```python
from build123d import *

# Parameters (mm, degrees)
SKETCH1_3_W         = 30
SKETCH1_3_H         = 31.716112931
SKETCH1_3_W_2       = 26.4
SKETCH1_3_H_2       = 26.4
BOSS_EXTRUDE3_DEPTH = 20
SKETCH1_10_W        = 26.4
SKETCH1_10_H        = 26.4
SKETCH1_10_R        = 10.5
BOSS_EXTRUDE7_DEPTH = 5
SKETCH1_R           = 10.5
CUT_EXTRUDE1_DEPTH  = 2
SKETCH2_R           = 1.4
CUT_EXTRUDE2_DEPTH  = 15


with BuildPart() as part:
    # Sketch1_3 → Boss-Extrude3 (new body)
    # profile 1 of 3: a face of its own
    with BuildSketch(Plane.XY):
        Polygon((-189.640703899, -24.770069728), (-175.564173506, -70.171428571), (-156.564173506, -70.171428571), (-159.640703899, -23.131847808), (-159.640703899, -1.887541502), (-189.640703899, -1.887541502), align=None)
    # profile 2 of 3: a face of its own
    with BuildSketch(Plane.XY):
        Polygon((-189.640703899, -24.770069728), (-175.564173506, -70.171428571), (-156.564173506, -70.171428571), (-159.640703899, -23.131847808), (-159.640703899, -1.887541502), (-189.640703899, -1.887541502), align=None)
    # profile 3 of 3: a face of its own
    with BuildSketch(Plane.XY):
        with Locations((-174.640703899, 13.970514963)):
            Rectangle(SKETCH1_3_W, SKETCH1_3_H)
        with Locations((-174.640703899, 14.828571429)):
            Rectangle(SKETCH1_3_W_2, SKETCH1_3_H_2, mode=Mode.SUBTRACT)
    extrude(amount=-BOSS_EXTRUDE3_DEPTH)

    # Sketch1_10 → Boss-Extrude7 (add)
    # profile 1 of 2: a face of its own
    with BuildSketch(Plane.XY):
        with Locations((-174.640703899, 14.828571429)):
            Rectangle(SKETCH1_10_W, SKETCH1_10_H)
        with Locations((-174.640703899, 14.828571429)):
            Circle(SKETCH1_10_R, mode=Mode.SUBTRACT)
    # profile 2 of 2: a face of its own
    with BuildSketch(Plane.XY):
        with Locations((-174.640703899, 14.828571429)):
            Circle(SKETCH1_10_R)
        with BuildLine():
            Line((-171.403251306, 11.018203899), (-167.861898306, 7.4768509))
            ThreePointArc((-167.861898306, 7.4768509), (-174.687644898, 4.828681602), (-181.488229417, 7.540814964))
            Line((-181.488229417, 7.540814964), (-177.949263698, 11.079780683))
            ThreePointArc((-177.949263698, 11.079780683), (-179.638278417, 14.672850745), (-178.176237805, 18.364105335))
            Line((-178.176237805, 18.364105335), (-177.949263698, 18.638938958))
            Line((-177.949263698, 18.638938958), (-181.456415012, 22.146090272))
            ThreePointArc((-181.456415012, 22.146090272), (-174.665862261, 24.828539781), (-167.861898306, 22.180291958))
            Line((-167.861898306, 22.180291958), (-171.403251306, 18.638938958))
            ThreePointArc((-171.403251306, 18.638938958), (-169.640703899, 14.828571429), (-171.403251306, 11.018203899))
        make_face(mode=Mode.SUBTRACT)
    extrude(amount=-BOSS_EXTRUDE7_DEPTH)

    # Sketch1 → Cut-Extrude1 (cut)
    with BuildSketch(Plane.XY):
        with Locations((-174.640703899, 14.828571429)):
            Circle(SKETCH1_R)
        with BuildLine():
            Line((-171.403251306, 11.018203899), (-167.861898306, 7.4768509))
            ThreePointArc((-167.861898306, 7.4768509), (-174.687644898, 4.828681602), (-181.488229417, 7.540814964))
            Line((-181.488229417, 7.540814964), (-177.949263698, 11.079780683))
            ThreePointArc((-177.949263698, 11.079780683), (-179.638278417, 14.672850745), (-178.176237805, 18.364105335))
            Line((-178.176237805, 18.364105335), (-177.949263698, 18.638938958))
            Line((-177.949263698, 18.638938958), (-181.456415012, 22.146090272))
            ThreePointArc((-181.456415012, 22.146090272), (-174.665862261, 24.828539781), (-167.861898306, 22.180291958))
            Line((-167.861898306, 22.180291958), (-171.403251306, 18.638938958))
            ThreePointArc((-171.403251306, 18.638938958), (-169.640703899, 14.828571429), (-171.403251306, 11.018203899))
        make_face(mode=Mode.SUBTRACT)
    extrude(amount=-CUT_EXTRUDE1_DEPTH, mode=Mode.SUBTRACT)

    # Sketch2 → Cut-Extrude2 (cut)
    with BuildSketch(Plane(origin=(0, -70.171428571, 0), x_dir=(-1, 0, 0), z_dir=(0, -1, 0))):
        with Locations(Location((161.564173506, 12, 0), (0, 0, 180))):
            Circle(SKETCH2_R)
        with Locations(Location((170.564173506, 12, 0), (0, 0, 180))):
            Circle(SKETCH2_R)
    extrude(amount=-CUT_EXTRUDE2_DEPTH, mode=Mode.SUBTRACT)


solid = part.part
```
Source: CAD feature listing. Evaluate the final solid. Frame: model axes, mm. A direction names the side the tool comes from. Round coordinates to 2 decimals unless told otherwise and drop trailing zeros. Loops run counter-clockwise (first coordinate to the right, second up) from the corner with the lowest first, then second, coordinate; pieces in that order, holes last. Notation, with made-up numbers: M 61.25,82 L 68.25,82 A23 cw 68.25,93 Z; hole C 43.25,47.25 d10. An arc over 180 degrees is marked long. Use a Markdown table: item, result. Add a question column.
1. Section query B-B on y = -62. Return the cut outline in (x, z), then the cut area to 3 significant figures.
2. Reachability of faces 1 (the flat face through (-179.68, 20.37, -3.48)), 2 (the flat face through (-158.08, -46.98, -9.86)), 3 (the flat face through (-175, 1.629, -12)), 4 (the flat face through (-166, -70.171, -10)), 5 (the cylindrical face through (-176.92, 4.58, -0.99)) from +Z, -Z, +X, -X, +Y, -Y: full face, straight path, thin tool, end or side. Return the list, or none.
3. Contact query for flat-ended pins moving along their axis: P1, Ø1.4, axis at x = -162, z = -12.5, coming from the -Y side; P2, Ø8, axis at y = -15, z = -11.5, coming from the +X side; P3, Ø1.5, axis at x = -163, y = 12.5, coming from the -Z side. Output: stop coordinate, or through.
4. Section query A-A on z = -12. Return the cut outline in (x, y), then the cut area to 3 significant figures.
5. Section query D-D on x = -183.5. Return the cut outline in (y, z), then the cut area to 3 significant figures.
6. Section query C-C on z = -19. Return the cut outline in (x, y), then the cut area to 3 significant figures.
7. Line query: line 1 (X direction, y = 3.5, z = -12.25); line 2 (Y direction, x = -171.5, z = -12.5); line 3 (Y direction, x = -174.5, z = -9.75). Output: solid intervals per line, ascending.
8. Mould query, pull axis Y, two halves, no side actions, for faces 6 (the flat face through (-175, 29.829, -10)), 7 (the flat face through (-181, 15, -5)), 8 (the cylindrical face through (-171.963, -62.776, -11.938)), 9 (the flat face through (-162, -55.171, -12)). Classes: pulls with the +Y half, pulls with the -Y half, needs draft (parallel to the pull), parting line crosses it, or undercut.
Reported:
| question | item | result |
|---|---|---|
| 1 | outline | M -178.1,-20 L -157.1,-20 L -157.1,0 L -178.1,0 Z; hole C -170.56,-12 d2.8; hole C -161.56,-12 d2.8 |
| 1 | area | 408 mm² |
| 2 | face 1 | +Z, -Z |
| 2 | face 2 | +Z, -Z, +X, +Y |
| 2 | face 3 | -Z |
| 2 | face 4 | +Z, -Z, +X, -X, -Y |
| 2 | face 5 | +Z |
| 3 | P1 | stops at y = -55.17 |
| 3 | P2 | stops at x = -159.64 |
| 3 | P3 | stops at z = -5 |
| 4 | outline | M -189.64,-24.77 L -175.56,-70.17 L -171.96,-70.17 L -171.96,-55.17 L -169.16,-55.17 L -169.16,-70.17 L -162.96,-70.17 L -162.96,-55.17 L -160.16,-55.17 L -160.16,-70.17 L -156.56,-70.17 L -159.64,-23.13 L -159.64,29.83 L -189.64,29.83 Z; hole M -187.84,1.63 L -161.44,1.63 L -161.44,28.03 L -187.84,28.03 Z |
| 4 | area | 1,970 mm² |
| 5 | outline | M -44.58,-20 L 1.63,-20 L 1.63,-5 L 28.03,-5 L 28.03,-20 L 29.83,-20 L 29.83,0 L 20.46,0 L 20.46,-2 L 9.19,-2 L 9.19,0 L -44.58,0 Z |
| 5 | area | 1,070 mm² |
| 6 | outline | M -189.64,-24.77 L -175.56,-70.17 L -156.56,-70.17 L -159.64,-23.13 L -159.64,29.83 L -189.64,29.83 Z; hole M -187.84,1.63 L -161.44,1.63 L -161.44,28.03 L -187.84,28.03 Z |
| 6 | area | 2,060 mm² |
| 7 | line 1 | x = -189.64 to -187.84, -161.44 to -159.64 |
| 7 | line 2 | y = -55.17 to 1.63, 28.03 to 29.83 |
| 7 | line 3 | y = -70.17 to 1.63, 28.03 to 29.83 |
| 8 | face 6 | pulls with the +Y half |
| 8 | face 7 | undercut |
| 8 | face 8 | needs draft |
| 8 | face 9 | pulls with the -Y half |
